Part model, mm, in its own coordinate system. Coordinates: 2 decimals unless noted, no trailing zeros. Loops run counter-clockwise (first coordinate to the right, second up) from the corner with the lowest first, then second, coordinate; pieces in that order, holes last. Notation, with made-up numbers: (33.5, 76.25) - (77.5, 76.25) arc R14 ccw to (77.5, 96.25) - close; hole circle Ø5 at (68, 25). An arc over 180 degrees is marked (long way). Use a Markdown table: item, result. Add a question column.
1. Drop a flat-ended pin along its axis: pin 1 (1.5 mm diameter, centred on x = 2, z = 3, fed in from +Y). Give the stop position or say it passes through.
2. Wall check: probe 1 along Y at (x, z) = (114.5, 0.55); probe 2 along X at (y, z) = (155.5, 0.25); probe 3 along Y at (x, z) = (4, 0.4). Give the ranges that are in metal, low to high. Write a range as [from, to].
3. Band-saw the part on C-C, the plane x = -4. Give the cut face in (y, z), plus the area to 3 significant figures.
4. Band-saw the part on A-A, the plane y = -160. Give the cut face in (x, z), plus the area to 3 significant figures.
5. Band-saw the part on B-B, the plane z = 1.45. Give the cut face in (x, y).
from build123d import *

# Parameters (mm, degrees)
SKETCH2_W           = 340
SKETCH2_H           = 340
BOSS_EXTRUDE1_DEPTH = 5
CHAMFER1_SIZE       = 5
CUT_EXTRUDE2_DEPTH  = 241.468293128
SKETCH5_W           = 50
SKETCH5_H           = 50
CUT_EXTRUDE3_DEPTH  = 241.468293128


with BuildPart() as part:
    # Sketch2 → Boss-Extrude1 (new body)
    with BuildSketch(Plane.XY):
        Rectangle(SKETCH2_W, SKETCH2_H)
    extrude(amount=BOSS_EXTRUDE1_DEPTH)

    # Chamfer1
    chamfer1_edges = [part.edges().sort_by_distance(p)[0] for p in [
        (170, -170, 2.5),
        (-170, -170, 2.5),
        (-170, 170, 2.5),
        (170, 170, 2.5),
    ]]
    chamfer(chamfer1_edges, length=CHAMFER1_SIZE)

    # Sketch4 → Cut-Extrude2 (cut, through all)
    with BuildSketch(Plane.XY.offset(5)):
        with BuildLine():
            Line((-7.8, 164.9), (7.8, 164.9))
            ThreePointArc((7.8, 164.9), (12.7, 160), (7.8, 155.1))
            Line((7.8, 155.1), (-7.8, 155.1))
            ThreePointArc((-7.8, 155.1), (-12.7, 160), (-7.8, 164.9))
        make_face()
        with BuildLine():
            Line((-117.8, -154.85), (-102.2, -154.85))
            ThreePointArc((-102.2, -154.85), (-97.05, -160), (-102.2, -165.15))
            Line((-102.2, -165.15), (-117.8, -165.15))
            ThreePointArc((-117.8, -165.15), (-122.95, -160), (-117.8, -154.85))
        make_face()
    cut_extrude2 = extrude(amount=-CUT_EXTRUDE2_DEPTH, mode=Mode.SUBTRACT)

    # Mirror1: Cut-Extrude2 across plane
    add(cut_extrude2.mirror(Plane(origin=(0, 0, 0), x_dir=(0, 0, 1), z_dir=(1, 0, 0))), mode=Mode.SUBTRACT)

    # Sketch5 → Cut-Extrude3 (cut, through all)
    with BuildSketch(Plane.XY.offset(5)):
        with Locations((0, 145)):
            Rectangle(SKETCH5_W, SKETCH5_H)
    extrude(amount=-CUT_EXTRUDE3_DEPTH, mode=Mode.SUBTRACT)


solid = part.part
Geometry check:
| question | item | result |
|---|---|---|
| 1 | pin 1 | stops at y = 120 |
| 2 | probe 1 | y = [-170, -165.15], [-154.85, 170] |
| 2 | probe 2 | x = [-170, -25], [25, 170] |
| 2 | probe 3 | y = [-170, 120] |
| 3 | outline | (-170, 0) - (120, 0) - (120, 5) - (-170, 5) - close |
| 3 | area | 1,450 mm^2 |
| 4 | outline | (-170, 0) - (-122.95, 0) - (-122.95, 5) - (-170, 5) - close; (-97.05, 0) - (97.05, 0) - (97.05, 5) - (-97.05, 5) - close; (122.95, 0) - (170, 0) - (170, 5) - (122.95, 5) - close |
| 4 | area | 1,440 mm^2 |
| 5 | outline | (-170, -165) - (-165, -170) - (165, -170) - (170, -165) - (170, 165) - (165, 170) - (25, 170) - (25, 120) - (-25, 120) - (-25, 170) - (-165, 170) - (-170, 165) - close; hole (-117.8, -165.15) - (-102.2, -165.15) arc R5.15 ccw to (-102.2, -154.85) - (-117.8, -154.85) arc R5.15 ccw to start; hole (102.2, -165.15) - (117.8, -165.15) arc R5.15 ccw to (117.8, -154.85) - (102.2, -154.85) arc R5.15 ccw to start |
